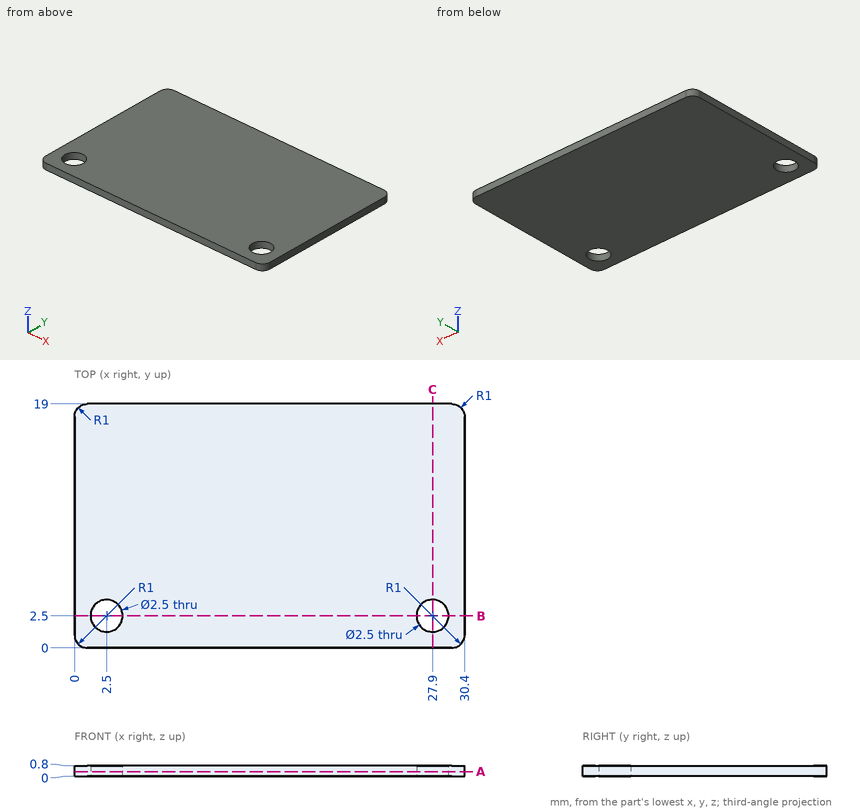
Print and shaded views of the part. All mm, measured from the part's lowest x, y and z. Coordinates: 2 decimals unless noted, no trailing zeros. Write each loop counter-clockwise with the first axis right and the second up, starting at its lowest first coordinate (ties: lowest second). Pieces come first, ordered by that corner, then holes. Notation, with made-up numbers: (-3, -25) - (44, -25) arc R22 cw to (44, -17) - close; hole circle Ø5 at (65, -32). An arc over 180 degrees is marked (long way). One line per question, with ' | ' between items. Start each with the question number.
Q1. Cut at C-C, the plane x = 27.9. List the corners of the cut face in (y, z), then the cut area to 3 significant figures.
Q2. Cut at B-B, the plane y = 2.5. List the corners of the cut face in (x, z), then the cut area to 3 significant figures.
Q3. Cut at A-A, the plane z = 0.35. List the corners of the cut face in (x, y).
Q4. Drill centre line: line 1 (Y direction, x = 27.9, z = 0.5). Where is it in solid material? Low to high. Write a range as [from, to].
Q5. Pin check, flat tip, straight feed: pin 1 (2 mm diameter, centred on x = 2.5, y = 2.5, fed in from +Z). Stop position of the tip, or through.
Answer below:
1) outline: (0, 0) - (1.25, 0) - (1.25, 0.8) - (0, 0.8) - close; (3.75, 0) - (19, 0) - (19, 0.8) - (3.75, 0.8) - close | area: 13.2 mm^2
2) outline: (0, 0) - (1.25, 0) - (1.25, 0.8) - (0, 0.8) - close; (3.75, 0) - (26.65, 0) - (26.65, 0.8) - (3.75, 0.8) - close; (29.15, 0) - (30.4, 0) - (30.4, 0.8) - (29.15, 0.8) - close | area: 20.3 mm^2
3) outline: (0, 1) arc R1 ccw to (1, 0) - (29.4, 0) arc R1 ccw to (30.4, 1) - (30.4, 18) arc R1 ccw to (29.4, 19) - (1, 19) arc R1 ccw to (0, 18) - close; hole circle Ø2.5 at (2.5, 2.5); hole circle Ø2.5 at (27.9, 2.5)
4) line 1: [0, 1.25], [3.75, 19]
5) pin 1: through
